Geometry check sheet. Reference: the model listing, model coordinates, mm. Face numbers are marked on the shaded views. A direction names the side the tool comes from. Round coordinates to 2 decimals unless told otherwise and drop trailing zeros. Write each loop counter-clockwise with the first axis right and the second up, starting at its lowest first coordinate (ties: lowest second). Pieces come first, ordered by that corner, then holes.
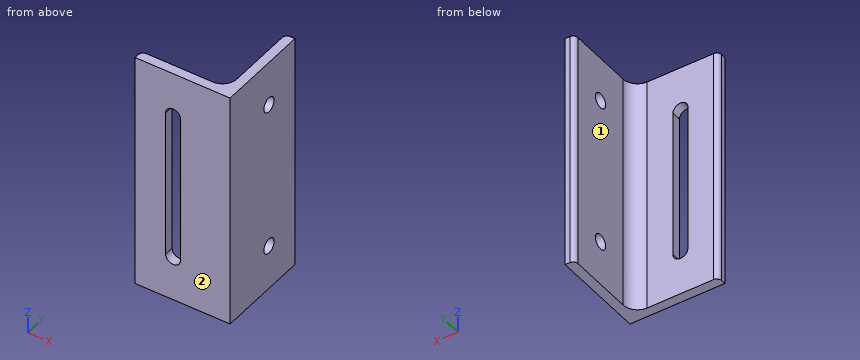
from build123d import *

# Parameters (mm, degrees)
BOSS_EXTRUDE1_DEPTH = 304.8
SKETCH3_W           = 34.414454966
SKETCH3_H           = 33.657940314
CUT_EXTRUDE1_DEPTH  = 529.6
SKETCH5_R           = 2.5
CUT_EXTRUDE2_DEPTH  = 101.6
CUT_EXTRUDE3_DEPTH  = 101.6


with BuildPart() as part:
    # Sketch2 → Boss-Extrude1 (new, symmetric)
    with BuildSketch(Plane.XY):
        with BuildLine():
            Line((-15.875, -15.875), (15.875, -15.875))
            Line((15.875, -15.875), (15.875, 15.875))
            Line((15.875, 15.875), (14.2875, 15.875))
            ThreePointArc((14.2875, 15.875), (13.164967985, 15.410032015), (12.7, 14.2875))
            Line((12.7, 14.2875), (12.7, -7.9248))
            ThreePointArc((12.7, -7.9248), (11.301376302, -11.301376302), (7.9248, -12.7))
            Line((7.9248, -12.7), (-14.2875, -12.7))
            ThreePointArc((-14.2875, -12.7), (-15.410032015, -13.164967985), (-15.875, -14.2875))
            Line((-15.875, -14.2875), (-15.875, -15.875))
        make_face()
    extrude(amount=BOSS_EXTRUDE1_DEPTH, both=True)

    # Sketch3 → Cut-Extrude1 (cut)
    with BuildSketch(Plane(origin=(0, 0, -304.8), x_dir=(-1, 0, 0), z_dir=(0, 0, -1))):
        with Locations((1.332227483, 0.953970157)):
            Rectangle(SKETCH3_W, SKETCH3_H)
    extrude(amount=-CUT_EXTRUDE1_DEPTH, mode=Mode.SUBTRACT)

    # Sketch5 → Cut-Extrude2 (cut)
    with BuildSketch(Plane.ZY.offset(-12.7)):
        with Locations(Location((289.8, 3.18135, 0), (0, 0, 270))):
            Circle(SKETCH5_R)
        with Locations(Location((239.8, 3.18135, 0), (0, 0, 270))):
            Circle(SKETCH5_R)
    extrude(amount=-CUT_EXTRUDE2_DEPTH, mode=Mode.SUBTRACT)

    # Sketch4 → Cut-Extrude3 (cut)
    with BuildSketch(Plane(origin=(0, -12.7, 0), x_dir=(1, 0, 0), z_dir=(0, 1, 0))):
        with BuildLine():
            Line((-0.68135, -239.8), (-0.68135, -289.8))
            ThreePointArc((-0.68135, -289.8), (-3.18135, -292.3), (-5.68135, -289.8))
            Line((-5.68135, -289.8), (-5.68135, -239.8))
            ThreePointArc((-5.68135, -239.8), (-3.18135, -237.3), (-0.68135, -239.8))
        make_face()
    extrude(amount=-CUT_EXTRUDE3_DEPTH, mode=Mode.SUBTRACT)


solid = part.part
1. Section check D-D (y = -2). Record the cut outline in (x, z) (3 decimals).
2. Access from +Z, -Z, +X, -X, +Y, -Y to the whole of each face (thin tool, end or side, straight path). Record for the marked faces 1 and 2.
3. Scan lines: line 1 along Y through (x, z) = (15.1, 289.8) (3 decimals); line 2 along X through (y, z) = (0, 298) (3 decimals); line 3 along Y through (x, z) = (2.5, 260) (3 decimals). Record each from-to range of solid material in increasing order.
4. Section check C-C (x = 13.5). Record the cut outline in (y, z) (3 decimals).
5. Section check B-B (z = 236.5). Record the cut outline in (x, y) (1 decimal).
6. Section check A-A (z = 257). Record the cut outline in (x, y) (1 decimal).
7. Depth check by flat-ended pin: pin 1 Ø12 at (x, z) = (-7.5, 282.5) entering from +Y; pin 2 Ø6 at (y, z) = (3.18, 289.8) entering from -X. Enter the tip coordinate at first touch or a pass-through.
Results below:
1. outline: (12.7, 224.8) - (15.875, 224.8) - (15.875, 304.8) - (12.7, 304.8) - close
2. face 1: +Z, -Z, -X, +Y
2. face 2: +Z, -Z, +X, -X, -Y
3. line 1: y = -15.875 to 0.681, 5.681 to 15.875
3. line 2: x = 12.7 to 15.875
3. line 3: y = -15.875 to -12.7
4. outline: (-15.875, 224.8) - (15.666, 224.8) - (15.666, 304.8) - (-15.875, 304.8) - close; hole circle Ø5 at (3.181, 239.8); hole circle Ø5 at (3.181, 289.8)
5. outline: (-15.9, -15.9) - (15.9, -15.9) - (15.9, 15.9) - (14.3, 15.9) arc R1.6 ccw to (12.7, 14.3) - (12.7, -7.9) arc R4.8 cw to (7.9, -12.7) - (-14.3, -12.7) arc R1.6 ccw to (-15.9, -14.3) - close
6. outline: (-15.9, -15.9) - (-5.7, -15.9) - (-5.7, -12.7) - (-14.3, -12.7) arc R1.6 ccw to (-15.9, -14.3) - close; (-0.7, -15.9) - (15.9, -15.9) - (15.9, 15.9) - (14.3, 15.9) arc R1.6 ccw to (12.7, 14.3) - (12.7, -7.9) arc R4.8 cw to (7.9, -12.7) - (-0.7, -12.7) - close
7. pin 1: stops at y = -12.7
7. pin 2: stops at x = 12.7
